```python
from build123d import *

# Parameters (mm, degrees)
F1_DEPTH = 25
F2_R     = 79.6498805285
F2_R_2   = 58.7498805617
F3_DEPTH = 50
F4_SIZE  = 5
F5_R     = 5


with BuildPart() as f1:
    # F0 (on Top) → F1 (new body)
    with BuildSketch(Plane.XY):
        with BuildLine():
            ThreePointArc((-58.7498805617, 0), (0, -58.7498805617), (58.7498805617, 0))
            ThreePointArc((58.7498805617, 0), (0, 58.7498805617), (-58.7498805617, 0))
        make_face()
        with BuildLine():
            Line((-28.5208848633, -7.3374048471), (-28.3221645254, -7.3374048471))
            add(Edge.make_bspline(
                [(-28.3221645254, -7.3374048471), (-26.118175323, -1.0957796878), (-25.2149010597, 0.656572383)],
                knots=[0, 0, 0, 1, 1, 1], degree=2))
            Line((-25.2149010597, 0.656572383), (-13.0206985053, 25.4966146234))
            Line((-13.0206985053, 25.4966146234), (-4.1053815266, 25.4966146234))
            Line((-4.1053815266, 25.4966146234), (-25.2149010597, -15.7739864662))
            Line((-25.2149010597, -15.7739864662), (-34.6450843684, -15.7739864662))
            Line((-34.6450843684, -15.7739864662), (-38.2310831936, 25.4966146234))
            Line((-38.2310831936, 25.4966146234), (-29.9028944861, 25.4966146234))
            Line((-29.9028944861, 25.4966146234), (-28.4666884075, 0.656572383))
            add(Edge.make_bspline(
                [(-28.4666884075, 0.656572383), (-28.3492627533, -0.6170443283), (-28.3492627533, -3.1010485523)],
                knots=[0, 0, 0, 1, 1, 1], degree=2))
            add(Edge.make_bspline(
                [(-28.3492627533, -3.1010485523), (-28.4034592091, -6.0095916801), (-28.5208848633, -7.3374048471)],
                knots=[0, 0, 0, 1, 1, 1], degree=2))
        make_face(mode=Mode.SUBTRACT)
        Polygon((6.9055317428, 15.786416293), (0.2122694519, -15.7739864662), (-8.278508623, -15.7739864662), (-1.5942790747, 15.786416293), align=None, mode=Mode.SUBTRACT)
        with BuildLine():
            add(Edge.make_bspline(
                [(21.836655315, 10.990029955), (25.7297673897, 16.3735445642), (30.7881032642, 16.3735445642)],
                knots=[0, 0, 0, 1, 1, 1], degree=2))
            add(Edge.make_bspline(
                [(30.7881032642, 16.3735445642), (34.9070339048, 16.3735445642), (37.2916779598, 13.3430594108)],
                knots=[0, 0, 0, 1, 1, 1], degree=2))
            add(Edge.make_bspline(
                [(37.2916779598, 13.3430594108), (39.6763220149, 10.3125742575), (39.6763220149, 4.8567977073)],
                knots=[0, 0, 0, 1, 1, 1], degree=2))
            add(Edge.make_bspline(
                [(39.6763220149, 4.8567977073), (39.6763220149, -0.5267169019), (37.7433150915, -5.5127908353)],
                knots=[0, 0, 0, 1, 1, 1], degree=2))
            add(Edge.make_bspline(
                [(37.7433150915, -5.5127908353), (35.810308168, -10.4988647686), (32.4501279086, -13.4209570104)],
                knots=[0, 0, 0, 1, 1, 1], degree=2))
            add(Edge.make_bspline(
                [(32.4501279086, -13.4209570104), (29.0899476492, -16.3430492521), (25.0523116923, -16.3430492521)],
                knots=[0, 0, 0, 1, 1, 1], degree=2))
            add(Edge.make_bspline(
                [(25.0523116923, -16.3430492521), (22.7128313504, -16.3430492521), (21.0191921067, -15.2952511067)],
                knots=[0, 0, 0, 1, 1, 1], degree=2))
            add(Edge.make_bspline(
                [(21.0191921067, -15.2952511067), (19.325552863, -14.2474529613), (17.8893467844, -11.7363505093)],
                knots=[0, 0, 0, 1, 1, 1], degree=2))
            Line((17.8893467844, -11.7363505093), (17.6635282186, -11.7363505093))
            add(Edge.make_bspline(
                [(17.6635282186, -11.7363505093), (17.3202839985, -16.2256235979), (16.4441079632, -20.0645392168)],
                knots=[0, 0, 0, 1, 1, 1], degree=2))
            Line((16.4441079632, -20.0645392168), (14.4117408708, -29.6663446356))
            Line((14.4117408708, -29.6663446356), (5.9119300532, -29.6663446356))
            Line((5.9119300532, -29.6663446356), (15.5679319278, 15.786416293))
            Line((15.5679319278, 15.786416293), (22.0624738808, 15.786416293))
            Line((22.0624738808, 15.786416293), (21.5837385213, 10.990029955))
            Line((21.5837385213, 10.990029955), (21.836655315, 10.990029955))
        make_face(mode=Mode.SUBTRACT)
        with BuildLine():
            add(Edge.make_bspline(
                [(4.0240868429, 19.7066265957), (-0.2393676798, 19.7066265957), (-0.2393676798, 23.1842325094)],
                knots=[0, 0, 0, 1, 1, 1], degree=2))
            add(Edge.make_bspline(
                [(-0.2393676798, 23.1842325094), (-0.2393676798, 25.6321057629), (1.1019946012, 26.8921733602)],
                knots=[0, 0, 0, 1, 1, 1], degree=2))
            add(Edge.make_bspline(
                [(1.1019946012, 26.8921733602), (2.4433568822, 28.1522409574), (4.9002628783, 28.1522409574)],
                knots=[0, 0, 0, 1, 1, 1], degree=2))
            add(Edge.make_bspline(
                [(4.9002628783, 28.1522409574), (6.9597281986, 28.1522409574), (8.0346245719, 27.2760649221)],
                knots=[0, 0, 0, 1, 1, 1], degree=2))
            add(Edge.make_bspline(
                [(8.0346245719, 27.2760649221), (9.1095209453, 26.3998888867), (9.1095209453, 24.7649624701)],
                knots=[0, 0, 0, 1, 1, 1], degree=2))
            add(Edge.make_bspline(
                [(9.1095209453, 24.7649624701), (9.1095209453, 22.5067768119), (7.8675188332, 21.1067017038)],
                knots=[0, 0, 0, 1, 1, 1], degree=2))
            add(Edge.make_bspline(
                [(7.8675188332, 21.1067017038), (6.6255167212, 19.7066265957), (4.0240868429, 19.7066265957)],
                knots=[0, 0, 0, 1, 1, 1], degree=2))
        make_face(mode=Mode.SUBTRACT)
    extrude(amount=F1_DEPTH)

    # F2 (on face) → F3 (join)
    with BuildSketch(Plane.XY.offset(25)):
        Circle(F2_R)
        Circle(F2_R_2, mode=Mode.SUBTRACT)
    extrude(amount=-F3_DEPTH)

    # F4
    f4_edges = [f1.edges().sort_by_distance(p)[0] for p in [
        (-79.649881, 0, 25),
    ]]
    chamfer(f4_edges, length=F4_SIZE)

    # F5
    f5_edges = [f1.edges().sort_by_distance(p)[0] for p in [
        (-58.749881, 0, -25),
    ]]
    fillet(f5_edges, radius=F5_R)


solid = f1.part
```
The listing builds one solid part. Answer for the finished solid, in the listing's coordinates (mm). A direction names the side the tool comes from. Coordinates: 2 decimals unless noted, no trailing zeros. Order: outer loops, then holes, each group sorted by start corner. A loop starts at its lowest first (then second) coordinate and runs counter-clockwise, first axis right, second up. Notation, with made-up numbers: M 79,5.5 L 131,5.5 A28 ccw 131,31.5 Z; hole C 29.25,24 d11. An arc over 180 degrees is marked long. Answer as a JSON object with one key per item and string values. Group by question number.
1. Section A-A on z = -16 is taken. Write down the section's boundary in (x, y).
2. Section B-B on z = 9 is taken. State how many separate pieces and enclosed holes the cut face has, then the cut area to 3 significant figures.
3. A tool of negligible diameter and unlimited length cuts with its end or side. For faces 1 (the flat face through (19, 15.786, 12)), 2 (the conical face through (-16.24, -73.11, 24.76)), 3 (the flat face through (12, 1, 0)), from which of +Z, -Z, +X, -X, +Y, -Y can it reach the whole face along a straight path? Write none if from no direction.
4. Flat-ended cylindrical pins translate along their axes: P1, Ø7.5, axis at x = -28.5, z = 14.5, coming from the +Y side; P2, Ø12, axis at x = -23.5, z = -15, coming from the +Y side; P3, Ø6, axis at x = 35.5, z = -8.5, coming from the +Y side. Find the tip coordinate at first contact, or state that the pin passes through.
5. Straight lines are drawn through the part: line 1 (Y direction, x = 0, z = -11.25); line 2 (X direction, y = -6, z = 4); line 3 (X direction, y = 10.5, z = 19). For each, find the intervals that lie inside material, in ascending order.
Values follow:
{
 "1": {"outline": "C 0,0 d159.3; hole C 0,0 d117.5"},
 "2": {"separate pieces": "1", "enclosed holes": "4", "area": "18,100 mm2"},
 "3": {"face 1": "+Z, -Z", "face 2": "+Z", "face 3": "-Z"},
 "4": {"P1": "y = 75.71", "P2": "y = 77.7", "P3": "y = 72.72"},
 "5": {"line 1": "-79.65 to -58.75, 58.75 to 79.65", "line 2": "-79.42 to -35.49, -28.44 to -27.85, -20.22 to -6.21, 2.29 to 10.94, 37.55 to 79.42", "line 3": "-78.95 to -36.93, -29.04 to -20.38, -11.78 to -2.71, 5.78 to 14.44, 38.83 to 78.95"}
}
